For this review, take the finished solid that the model builds, in its own axes (mm). Face numbers are marked on the shaded views. A direction names the side the tool comes from. Give positions to 0.01 mm unless a question says otherwise; leave off trailing zeros. Write each loop counter-clockwise with the first axis right and the second up, starting at its lowest first coordinate (ties: lowest second). Pieces come first, ordered by that corner, then holes. Notation, with made-up numbers: (29.5, 34.25) -> (41.5, 34.25) arc R23 ccw to (41.5, 52.25) -> close; hole circle Ø2 at (61.25, 57). An arc over 180 degrees is marked (long way). Write item = value, one per line.
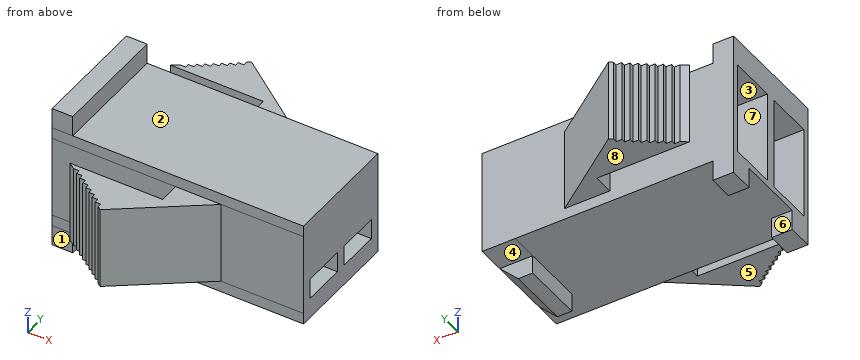
```python
from build123d import *

# Parameters (mm, degrees)
F1_DEPTH  = 5.1
F2_W      = 3.345763
F2_H      = 0.55
F2_W_2    = 3.297828
F3_DEPTH  = 15
F5_DEPTH  = 25
F6_DEPTH  = 10
F7_W      = 5.7
F7_H      = 1
F7_W_2    = 1.2
F8_DEPTH  = 1
F11_DEPTH = 5.7
F12_W     = 1.586434
F12_H     = 1.404738
F12_W_2   = 1.617856
F12_H_2   = 1.427827
F13_DEPTH = 3
F14_W     = 2.1
F14_H     = 1
F15_DEPTH = 3
F16_W     = 2.3
F16_H     = 4.5
F17_DEPTH = 5


with BuildPart() as f1:
    # F0 (on Top) → F1 (new body)
    with BuildSketch(Plane.XY):
        Polygon((-0.1, 2.85), (-6.1, 2.85), (-6.1, -2.85), (-0.1, -2.85), (-0.1, -3.85), (-4.6, -3.85), (-1.9, -5.8), (2.1, -2.85), (6.1, -2.85), (6.1, 2.85), (2.1, 2.85), (-1.9, 5.8), (-4.6, 3.85), (-0.1, 3.85), align=None)
    extrude(amount=F1_DEPTH)

    # F2 (on face) → F3 (cut)
    with BuildSketch(Plane.YZ.offset(6.1)):
        with Locations((-4.522881, 4.825)):
            Rectangle(F2_W, F2_H)
        with Locations((-4.522881, 0.275)):
            Rectangle(F2_W, F2_H)
        with Locations((4.498914, 4.825)):
            Rectangle(F2_W_2, F2_H)
        with Locations((4.498914, 0.275)):
            Rectangle(F2_W_2, F2_H)
    extrude(amount=-F3_DEPTH, mode=Mode.SUBTRACT)

    # F4 (on face) → F5 (cut)
    with BuildSketch(Plane.XY.offset(4.55)):
        Polygon((-4.011046, 4.075356), (-4.011046, 4.275356), (-4.287969, 4.075356), align=None)
        Polygon((-3.734123, 4.275356), (-3.734123, 4.475356), (-4.011046, 4.275356), align=None)
        Polygon((-3.4572, 4.475356), (-3.4572, 4.675356), (-3.734123, 4.475356), align=None)
        Polygon((-3.180277, 4.675356), (-3.180277, 4.875356), (-3.4572, 4.675356), align=None)
        Polygon((-2.903354, 4.875356), (-2.903354, 5.075356), (-3.180277, 4.875356), align=None)
        Polygon((-2.626431, 5.075356), (-2.626431, 5.275356), (-2.903354, 5.075356), align=None)
        Polygon((-2.349508, 5.275356), (-2.349508, 5.475356), (-2.626431, 5.275356), align=None)
        Polygon((-2.349508, 5.475356), (-2.072585, 5.475356), (-2.072585, 5.675356), align=None)
        Polygon((-3.734123, -4.475356), (-3.4572, -4.675356), (-3.4572, -4.475356), align=None)
        Polygon((-2.072585, -5.475356), (-2.349508, -5.475356), (-2.072585, -5.675356), align=None)
        Polygon((-2.349508, -5.275356), (-2.626431, -5.275356), (-2.349508, -5.475356), align=None)
        Polygon((-2.626431, -5.075356), (-2.903354, -5.075356), (-2.626431, -5.275356), align=None)
        Polygon((-2.903354, -4.875356), (-3.180277, -4.875356), (-2.903354, -5.075356), align=None)
        Polygon((-3.180277, -4.675356), (-3.4572, -4.675356), (-3.180277, -4.875356), align=None)
        Polygon((-4.287969, -4.075356), (-4.011046, -4.275356), (-4.011046, -4.075356), align=None)
        Polygon((-4.011046, -4.275356), (-3.734123, -4.475356), (-3.734123, -4.275356), align=None)
    extrude(amount=-F5_DEPTH, mode=Mode.SUBTRACT)

    # F4 (on face) → F6 (cut)
    with BuildSketch(Plane.XY.offset(4.55)):
        Polygon((-4.011046, 4.075356), (-4.011046, 4.275356), (-4.287969, 4.075356), align=None)
        Polygon((-3.734123, 4.275356), (-3.734123, 4.475356), (-4.011046, 4.275356), align=None)
        Polygon((-3.4572, 4.475356), (-3.4572, 4.675356), (-3.734123, 4.475356), align=None)
        Polygon((-3.180277, 4.675356), (-3.180277, 4.875356), (-3.4572, 4.675356), align=None)
        Polygon((-2.903354, 4.875356), (-2.903354, 5.075356), (-3.180277, 4.875356), align=None)
        Polygon((-2.626431, 5.075356), (-2.626431, 5.275356), (-2.903354, 5.075356), align=None)
        Polygon((-2.349508, 5.275356), (-2.349508, 5.475356), (-2.626431, 5.275356), align=None)
        Polygon((-2.349508, 5.475356), (-2.072585, 5.475356), (-2.072585, 5.675356), align=None)
        Polygon((-3.734123, -4.475356), (-3.4572, -4.675356), (-3.4572, -4.475356), align=None)
        Polygon((-2.072585, -5.475356), (-2.349508, -5.475356), (-2.072585, -5.675356), align=None)
        Polygon((-2.349508, -5.275356), (-2.626431, -5.275356), (-2.349508, -5.475356), align=None)
        Polygon((-2.626431, -5.075356), (-2.903354, -5.075356), (-2.626431, -5.275356), align=None)
        Polygon((-2.903354, -4.875356), (-3.180277, -4.875356), (-2.903354, -5.075356), align=None)
        Polygon((-3.180277, -4.675356), (-3.4572, -4.675356), (-3.180277, -4.875356), align=None)
        Polygon((-4.287969, -4.075356), (-4.011046, -4.275356), (-4.011046, -4.075356), align=None)
        Polygon((-4.011046, -4.275356), (-3.734123, -4.475356), (-3.734123, -4.275356), align=None)
    extrude(amount=-F6_DEPTH, mode=Mode.SUBTRACT)


with BuildPart() as f8:
    # F7 (on face) → F8 (new body)
    with BuildSketch(Plane(origin=(-6.1, 0, 0), x_dir=(0, -1, 0), z_dir=(-1, 0, 0))):
        with Locations((0, 5.6)):
            Rectangle(F7_W, F7_H)
        with Locations((-2.25, -0.5)):
            Rectangle(F7_W_2, F7_H)
        with Locations((2.25, -0.5)):
            Rectangle(F7_W_2, F7_H)
    extrude(amount=-F8_DEPTH)


with BuildPart() as f1_1:
    add(f1.part)

    # F9: union F8
    add(f8.part)

    # F10 (on face) → F11 (join, through all)
    with BuildSketch(Plane(origin=(0, 2.85, 0), x_dir=(-1, 0, 0), z_dir=(0, 1, 0))):
        Polygon((-6.1, 0), (-5.2, -0.9), (-4.5, -0.9), (-4.5, 0), align=None)
    extrude(amount=-F11_DEPTH)

    # F12 (on face) → F13 (cut)
    with BuildSketch(Plane(origin=(4.5, 0, 0), x_dir=(0, -1, 0), z_dir=(-1, 0, 0))):
        with Locations((2.293217, -0.702369)):
            Rectangle(F12_W, F12_H)
        with Locations((-2.308928, -0.713913)):
            Rectangle(F12_W_2, F12_H_2)
    extrude(amount=-F13_DEPTH, mode=Mode.SUBTRACT)

    # F14 (on face) → F15 (cut)
    with BuildSketch(Plane.YZ.offset(6.1)):
        with Locations((-1.3, 1.5)):
            Rectangle(F14_W, F14_H)
        with Locations((1.3, 1.5)):
            Rectangle(F14_W, F14_H)
    extrude(amount=-F15_DEPTH, mode=Mode.SUBTRACT)

    # F16 (on face) → F17 (cut)
    with BuildSketch(Plane(origin=(-6.1, 0, 0), x_dir=(0, -1, 0), z_dir=(-1, 0, 0))):
        with Locations((-1.4, 2.55)):
            Rectangle(F16_W, F16_H)
        with Locations((1.4, 2.55)):
            Rectangle(F16_W, F16_H)
    extrude(amount=-F17_DEPTH, mode=Mode.SUBTRACT)


solid = f1_1.part
```
(1) Take a section at C-C (x = 2.75). Write out the cut boundary in (y, z).
Answers below:
outline = (-2.85, 0) -> (2.85, 0) -> (2.85, 5.1) -> (-2.85, 5.1) -> close
(2) Take a section at A-A (x = 4.25). Write out the cut boundary in (y, z), plus the area to 3 significant figures.
Answers below:
outline = (-2.85, 0) -> (2.85, 0) -> (2.85, 5.1) -> (-2.85, 5.1) -> close; hole (-2.35, 1) -> (-0.25, 1) -> (-0.25, 2) -> (-2.35, 2) -> close; hole (0.25, 1) -> (2.35, 1) -> (2.35, 2) -> (0.25, 2) -> close
area = 24.9 mm^2
(3) To check wall thickness, follow probe 1 along Y at (x, z) = (-4.75, 0.75); probe 2 along Y at (x, z) = (-2.25, 3.5); probe 3 along Z at (x, y) = (-3.25, -1.25). State the ranges of each line that lie inside material, in increasing order.
Answers below:
probe_1 = -2.85 to -2.55, -0.25 to 0.25, 2.55 to 2.85
probe_2 = -5.48 to -3.85, -2.85 to -2.55, -0.25 to 0.25, 2.55 to 2.85, 3.85 to 5.48
probe_3 = 0 to 0.3, 4.8 to 5.1
(4) Tool access review of the marked faces 4, 5, 6, 7 and 8: name each direction out of +Z, -Z, +X, -X, +Y, -Y from which nothing blocks a thin tool from reaching the whole face with its end or side.
Answers below:
face_4 = -Z, +X, +Y
face_5 = -Z, +X, -X, -Y
face_6 = -Z, +X, -X
face_7 = -X
face_8 = -Z, +X, -X, +Y
(5) The part is to be moulded in two halves that separate along Y. For the marked faces 1, 2 and 3, say which applies: released by +Y, released by -Y, zero draft, split by the parting line, or undercut.
Answers below:
face_1 = released by -Y
face_2 = zero draft
face_3 = undercut
(6) Take a section at B-B (y = -0.5). Write out the cut boundary in (x, z), plus the area to 3 significant figures.
Answers below:
outline = (-6.1, 0) -> (4.5, 0) -> (4.5, -0.9) -> (5.2, -0.9) -> (6.1, 0) -> (6.1, 1) -> (3.1, 1) -> (3.1, 2) -> (6.1, 2) -> (6.1, 5.1) -> (-5.1, 5.1) -> (-5.1, 6.1) -> (-6.1, 6.1) -> (-6.1, 4.8) -> (-1.1, 4.8) -> (-1.1, 0.3) -> (-6.1, 0.3) -> close
area = 38.8 mm^2
(7) For pin 1 (0.7 mm diameter, centred on x = -4.5, y = 1.5, fed in from -Z); pin 2 (1 mm diameter, centred on x = -3, z = 4.5, fed in from +Y); pin 3 (0.6 mm diameter, centred on x = -2, z = 0, fed in from -Y), all flat-tipped, find the tip position at first contact; note any pin that passes through.
Answers below:
pin_1 = 0
pin_2 = 5.28
pin_3 = -2.85
(8) Take a section at D-D (x = 1). Write out the cut boundary in (y, z), plus the area to 3 significant figures.
Answers below:
outline = (-3.66, 0.55) -> (-2.85, 0.55) -> (-2.85, 0) -> (2.85, 0) -> (2.85, 0.55) -> (3.66, 0.55) -> (3.66, 4.55) -> (2.85, 4.55) -> (2.85, 5.1) -> (-2.85, 5.1) -> (-2.85, 4.55) -> (-3.66, 4.55) -> close
area = 35.6 mm^2
